Here's the drawing with two shaded views (mm, measured from the low corner). I have some questions. Give positions to 0.01 mm unless a question says otherwise; leave off trailing zeros. Loops run counter-clockwise (first coordinate to the right, second up) from the corner with the lowest first, then second, coordinate; pieces in that order, holes last. Notation, with made-up numbers: (86, -9.5) - (107, -9.5) arc R12 cw to (107, 9.5) - close; hole circle Ø4 at (16, -6.75). An arc over 180 degrees is marked (long way). Write each question's results on one line, items separated by ' | '. Start each with the question number.
1) I want a section at C-C, the plane y = 7.5. Write out the boundary of the cut face in (x, z).
2) I'm going to push flat-ended pins straight in: pin 1 (2 mm diameter, centred on x = 2.5, z = 14, fed in from -Y) (1 decimal); pin 2 (8 mm diameter, centred on x = 6.5, y = 8, fed in from +Z); pin 3 (2 mm diameter, centred on x = 8.5, y = 9.5, fed in from +Z) (1 decimal); pin 4 (2.5 mm diameter, centred on x = 7.5, y = 7.5, fed in from -Z). Where does each tip first touch, or does it pass through?
3) I want a section at D-D, the plane z = 25.5. Write out the boundary of the cut face in (x, y) (1 decimal).
4) I want a section at B-B, the plane x = 12. Write out the boundary of the cut face in (y, z).
5) I want a section at A-A, the plane z = 9.5. Write out the boundary of the cut face in (x, y).
6) If we mould it in two halves opening along X, with no side actions, what happens to the marked faces 1, 2 and 3? For each: +X half, -X half, draft (parallel to the pull), parting line (faces both ways), or undercut.
7) If I drill on probe 1 along X at (y, z) = (7.5, 11); probe 2 along Y at (x, z) = (2, 29.5), over which ranges is the centre line in solid material (lowest first)? Write a range as [from, to].
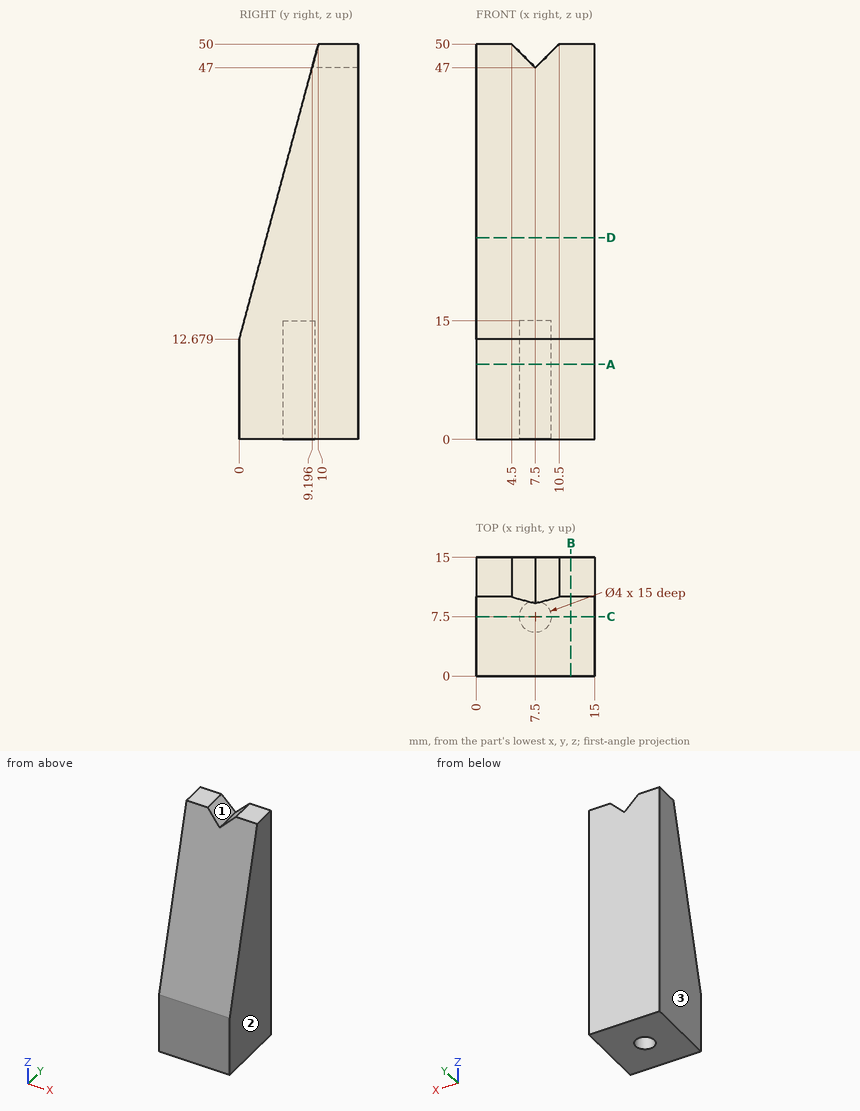
Answers:
1) outline: (0, 0) - (5.5, 0) - (5.5, 15) - (9.5, 15) - (9.5, 0) - (15, 0) - (15, 40.67) - (0, 40.67) - close
2) pin 1: stops at y = 0.1 | pin 2: stops at z = 50 | pin 3: stops at z = 49 | pin 4: stops at z = 15
3) outline: (0, 3.4) - (15, 3.4) - (15, 15) - (0, 15) - close
4) outline: (0, 0) - (15, 0) - (15, 50) - (10, 50) - (0, 12.68) - close
5) outline: (0, 0) - (15, 0) - (15, 15) - (0, 15) - close; hole circle Ø4 at (7.5, 7.5)
6) face 1: undercut | face 2: +X half | face 3: -X half
7) probe 1: x = [0, 5.5], [9.5, 15] | probe 2: y = [4.51, 15]
